from build123d import *

# Parameters (mm, degrees)
ESQUISSE1_W             = 10
ESQUISSE1_H             = 20
ESQUISSE1_W_2           = 81
ESQUISSE1_H_2           = 50
BOSS_EXTRU_1_DEPTH      = 6
ESQUISSE2_R             = 1.4
ENL_V_MAT_EXTRU_1_DEPTH = 6
ESQUISSE3_R             = 3
ENL_V_MAT_EXTRU_2_DEPTH = 4


with BuildPart() as part:
    # Esquisse1 → Boss.-Extru.1 (new body)
    with BuildSketch(Plane.XY):
        with Locations((-5, 25)):
            Rectangle(ESQUISSE1_W, ESQUISSE1_H)
        with Locations((40.5, 25)):
            Rectangle(ESQUISSE1_W_2, ESQUISSE1_H_2)
        with Locations((86, 25)):
            Rectangle(ESQUISSE1_W, ESQUISSE1_H)
    extrude(amount=BOSS_EXTRU_1_DEPTH)

    # Esquisse2 → Enlèv. mat.-Extru.1 (cut)
    with BuildSketch(Plane(origin=(0, 0, 0), x_dir=(-1, 0, 0), z_dir=(0, 0, -1))):
        with Locations((-44.550340057, 16.065313345)):
            Circle(ESQUISSE2_R)
        with Locations((-44.550340057, 28.065313345)):
            Circle(ESQUISSE2_R)
        with Locations((-68.550340057, 28.065313345)):
            Circle(ESQUISSE2_R)
        with Locations((-68.550340057, 16.065313345)):
            Circle(ESQUISSE2_R)
    extrude(amount=-ENL_V_MAT_EXTRU_1_DEPTH, mode=Mode.SUBTRACT)

    # Esquisse3 → Enlèv. mat.-Extru.2 (cut)
    with BuildSketch(Plane(origin=(0, 0, 0), x_dir=(-1, 0, 0), z_dir=(0, 0, -1))):
        with Locations((-68.550340057, 28.065313345)):
            Circle(ESQUISSE3_R)
        with Locations((-44.550340057, 28.065313345)):
            Circle(ESQUISSE3_R)
        with Locations((-44.550340057, 16.065313345)):
            Circle(ESQUISSE3_R)
        with Locations((-68.550340057, 16.065313345)):
            Circle(ESQUISSE3_R)
    extrude(amount=-ENL_V_MAT_EXTRU_2_DEPTH, mode=Mode.SUBTRACT)


solid = part.part
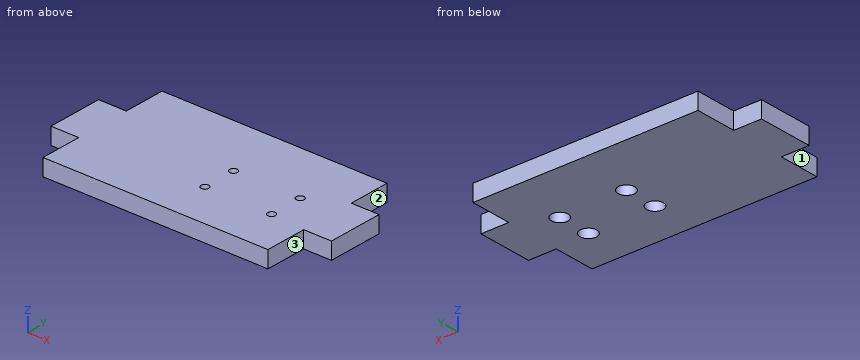
Input: part model. Units: mm. Frame: model coordinates. Face numbers are marked on the shaded views. A direction names the side the tool comes from. Round coordinates to 2 decimals unless told otherwise and drop trailing zeros. Write each loop counter-clockwise with the first axis right and the second up, starting at its lowest first coordinate (ties: lowest second). Pieces come first, ordered by that corner, then holes.
1) Cut plane B-B (x = -1.5). Return the cut outline in (y, z).
2) Ray query, L1, parallel to Y at x = -3, z = 4.5; L2, parallel to X at y = 13.5, z = 3.55; L3, parallel to X at y = 47.5, z = 0.65. Return the intervals inside material, ascending.
3) Cut plane C-C (y = 42.5). Return the cut outline in (x, z).
4) Reachability of the marked faces 1, 2 and 3 from +Z, -Z, +X, -X, +Y, -Y: full face, straight path, thin tool, end or side. Return the list, or none.
5) Cut plane A-A (z = 1.15). Return the cut outline in (x, y).
6) Contact query for flat-ended pins moving along their axis: P1, Ø1.8, axis at x = -3.5, z = 1.5, coming from the -Y side; P2, Ø1.8, axis at x = -4.5, z = 3, coming from the +Y side; P3, Ø1.8, axis at x = 68.5, y = 26.5, coming from the -Z side. Output: stop coordinate, or through.
Geometry says:
1. outline: (15, 0) - (35, 0) - (35, 6) - (15, 6) - close
2. L1: y = 15 to 35
2. L2: x = 0 to 42.99, 46.11 to 66.99, 70.11 to 81
2. L3: x = 0 to 81
3. outline: (0, 0) - (81, 0) - (81, 6) - (0, 6) - close
4. face 1: +Z, -Z, -X, -Y
4. face 2: +Z, -Z, +X, +Y
4. face 3: +Z, -Z, +X, -Y
5. outline: (-10, 15) - (0, 15) - (0, 0) - (81, 0) - (81, 15) - (91, 15) - (91, 35) - (81, 35) - (81, 50) - (0, 50) - (0, 35) - (-10, 35) - close; hole circle Ø6 at (44.55, 16.07); hole circle Ø6 at (44.55, 28.07); hole circle Ø6 at (68.55, 16.07); hole circle Ø6 at (68.55, 28.07)
6. P1: stops at y = 15
6. P2: stops at y = 35
6. P3: stops at z = 4
